```python
from build123d import *

# Parameters (mm, degrees)
SKETCH_W     = 40
SKETCH_H     = 40
PAD_DEPTH    = 10
SKETCH001_W  = 35
SKETCH001_H  = 35
POCKET_DEPTH = 5
FILLET_R     = 1
FILLET001_R  = 1
FILLET002_R  = 1
FILLET003_R  = 1
FILLET004_R  = 1
SKETCH002_R  = 1.5
HOLE_DEPTH   = 25


with BuildPart() as part:
    # Sketch → Pad (new body)
    with BuildSketch(Plane.XY):
        Rectangle(SKETCH_W, SKETCH_H)
    extrude(amount=PAD_DEPTH)

    # Sketch001 (on Face6 of Pad) → Pocket (cut)
    with BuildSketch(Plane.XY.offset(10)):
        Rectangle(SKETCH001_W, SKETCH001_H)
    extrude(amount=-POCKET_DEPTH, mode=Mode.SUBTRACT)

    # Fillet
    fillet_edges = [part.edges().sort_by_distance(p)[0] for p in [
        (-20, -20, 5),
    ]]
    fillet(fillet_edges, radius=FILLET_R)

    # Fillet001
    fillet001_edges = [part.edges().sort_by_distance(p)[0] for p in [
        (20, -20, 5),
    ]]
    fillet(fillet001_edges, radius=FILLET001_R)

    # Fillet002
    fillet002_edges = [part.edges().sort_by_distance(p)[0] for p in [
        (20, 20, 5),
    ]]
    fillet(fillet002_edges, radius=FILLET002_R)

    # Fillet003
    fillet003_edges = [part.edges().sort_by_distance(p)[0] for p in [
        (-20, 20, 5),
    ]]
    fillet(fillet003_edges, radius=FILLET003_R)

    # Fillet004
    fillet004_edges = [part.edges().sort_by_distance(p)[0] for p in [
        (-20, 0, 10),
    ]]
    fillet(fillet004_edges, radius=FILLET004_R)

    # Sketch002 (on Face23 of Fillet004) → Hole (cut)
    with BuildSketch(Plane.XY.offset(5)):
        with Locations((-15, 15)):
            Circle(SKETCH002_R)
        with Locations((15, 15)):
            Circle(SKETCH002_R)
        with Locations((-15, -15)):
            Circle(SKETCH002_R)
        with Locations((15, -15)):
            Circle(SKETCH002_R)
    extrude(amount=-HOLE_DEPTH, mode=Mode.SUBTRACT)


solid = part.part
```
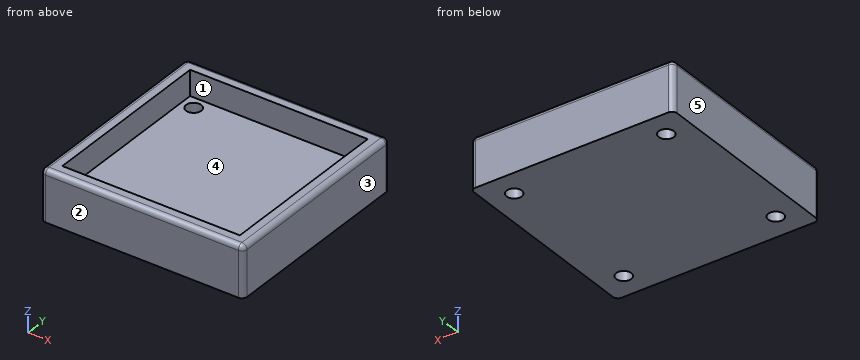
Design review of the part built by this model. Coordinates are the model's own, in mm. Face numbers are marked on the shaded views. A direction names the side the tool comes from. Round coordinates to 2 decimals unless told otherwise and drop trailing zeros. Write each loop counter-clockwise with the first axis right and the second up, starting at its lowest first coordinate (ties: lowest second). Pieces come first, ordered by that corner, then holes. Notation, with made-up numbers: (18, -18.75) -> (69, -18.75) arc R22 ccw to (69, 5.25) -> close; hole circle Ø7 at (42, 10). An arc over 180 degrees is marked (long way). Write item = value, one per line. Start each with the question number.
1) Mouldability with a two-part tool opening along X and no side actions: class the marked faces 1, 2 and 3 as +X half, -X half, draft (parallel to the pull), parting line (faces both ways), or undercut.
2) Take a section at A-A, the plane y = 15. State the section outline as (x, z) points, plus the area to 3 significant figures.
3) Tool access review of the marked faces 4 and 5: name each direction out of +Z, -Z, +X, -X, +Y, -Y from which nothing blocks a thin tool from reaching the whole face with its end or side.
4) Wall thickness on probe 1 along Y at (x, z) = (15, 3.7); probe 2 along X at (y, z) = (-3, 8.75): over which ranges is each line inside the solid? List them lowest first. Write a range as from..to.
5) Clearance check with a flat-ended pin moving along its axis: pin 1 (2 mm diameter, centred on x = 11, y = -11, fed in from +Z). State where the tip first meets the part, or that it passes through.
6) Take a section at D-D, the plane z = 2.75. State the section outline as (x, y) points, plus the area to 3 significant figures.
7) Take a section at C-C, the plane z = 5.5. State the section outline as (x, y) points.
Results list:
q1.face_1 = undercut
q1.face_2 = draft
q1.face_3 = +X half
q2.outline = (-20, 0) -> (-16.5, 0) -> (-16.5, 5) -> (-17.5, 5) -> (-17.5, 10) -> (-19, 10) arc R1 ccw to (-20, 9) -> close; (-13.5, 0) -> (13.5, 0) -> (13.5, 5) -> (-13.5, 5) -> close; (16.5, 0) -> (20, 0) -> (20, 9) arc R1 ccw to (19, 10) -> (17.5, 10) -> (17.5, 5) -> (16.5, 5) -> close
q2.area = 195 mm²
q3.face_4 = +Z
q3.face_5 = +Z, -Z, -X, +Y, -Y
q4.probe_1 = -20..-16.5, -13.5..13.5, 16.5..20
q4.probe_2 = -20..-17.5, 17.5..20
q5.pin_1 = 5
q6.outline = (-20, -19) arc R1 ccw to (-19, -20) -> (19, -20) arc R1 ccw to (20, -19) -> (20, 19) arc R1 ccw to (19, 20) -> (-19, 20) arc R1 ccw to (-20, 19) -> close; hole circle Ø3 at (-15, -15); hole circle Ø3 at (-15, 15); hole circle Ø3 at (15, -15); hole circle Ø3 at (15, 15)
q6.area = 1,570 mm²
q7.outline = (-20, -19) arc R1 ccw to (-19, -20) -> (19, -20) arc R1 ccw to (20, -19) -> (20, 19) arc R1 ccw to (19, 20) -> (-19, 20) arc R1 ccw to (-20, 19) -> close; hole (-17.5, -17.5) -> (17.5, -17.5) -> (17.5, 17.5) -> (-17.5, 17.5) -> close
